Build history of the part. All positions in model axes, mm. A direction names the side the tool comes from. Round coordinates to 2 decimals unless told otherwise and drop trailing zeros. Write each loop counter-clockwise with the first axis right and the second up, starting at its lowest first coordinate (ties: lowest second). Pieces come first, ordered by that corner, then holes. Notation, with made-up numbers: (79.25, 43) - (137.25, 43) arc R29 cw to (137.25, 75) - close; hole circle Ø4 at (50.5, 83). An arc over 180 degrees is marked (long way). Answer as a JSON object with one key per item and string values. Group by question number.
Item 1: Slice it at C-C, the plane x = 49. List the corners of the cut face in (y, z).
Item 2: Slice it at B-B, the plane z = 36.22. List the corners of the cut face in (x, y).
Item 3: Slice it at A-A, the plane x = 10. List the corners of the cut face in (y, z).
Item 4: Slice it at D-D, the plane y = 21.75. List the corners of the cut face in (x, z), then the cut area to 4 significant figures.
Item 5: Probe line 1 (Z direction, x = 10, y = 10.75); line 2 (Z direction, x = 75.5, y = 4.75); line 3 (X direction, y = 27, z = -70). List the from-to ranges inside material, lowest first. Write a range as from..to.
Item 6: Which spindle directions (+Z, -Z, +X, -X, +Y, -Y) get a long thin tool onto all of the face, cutting with end or side? Do faces 4 (the flat face through (44, 15, 22)), 5 (the cylindrical face through (86.787, 3.252, -40.49)), 6 (the cylindrical face through (89.248, 15.21, -79.287)). Say none if no direction does.
Item 7: Flat gauge pins, fed straight in: pin 1 (7.5 mm diameter, centred on x = 36, y = 20, fed in from +Z); pin 2 (3 mm diameter, centred on x = 79, z = 14.5, fed in from +Y); pin 3 (5 mm diameter, centred on x = 56, z = -48.5, fed in from +Y). Where does each tip first touch, or does it go through?
Item 8: Two-plate mould, pull along Z, no slides. Class faces 1 (the flat face through (44, 16, -80)), 2 (the flat face through (0, 11, -32)), 3 (the cylindrical face through (45.56, 3.252, -76.787)): +Z half, -Z half, draft (parallel to the pull), parting line (faces both ways), or undercut.
from build123d import *

# Parameters (mm, degrees)
BOSS_EXTRUDE1_DEPTH    = 90
SHELL1_T               = -2.5
SKETCH2_W              = 90
SKETCH2_H              = 45
BOSS_EXTRUDE2_DEPTH    = 15
F_10_0MM_DOWEL_HOLE1_D = 10
FILLET1_R              = 2.5


with BuildPart() as part:
    # Sketch1 → Boss-Extrude1 (new body)
    with BuildSketch(Plane(origin=(0, 0, 0), x_dir=(0, 0, -1), z_dir=(1, 0, 0))):
        Polygon((0, 0), (80, 0), (80, 30), (0, 15), align=None)
    extrude(amount=BOSS_EXTRUDE1_DEPTH)

    # Shell1
    shell1_openings = [part.faces().sort_by_distance(p)[0] for p in [
        (45, 22.5, -40),
    ]]
    offset(amount=SHELL1_T, openings=shell1_openings, kind=Kind.INTERSECTION)

    # Sketch2 → Boss-Extrude2 (add)
    with BuildSketch(Plane.XZ):
        with Locations((45, 22.5)):
            Rectangle(SKETCH2_W, SKETCH2_H)
    extrude(amount=-BOSS_EXTRUDE2_DEPTH)

    # Ø10.0mm Dowel Hole1 (through all)
    with Locations(Plane.XZ):
        with Locations((10, 36.22)):
            Hole(F_10_0MM_DOWEL_HOLE1_D / 2)

    # Fillet1
    fillet1_edges = [part.edges().sort_by_distance(p)[0] for p in [
        (90, 15, -80),
        (2.5, 8.984375, -2.5),
        (2.5, 2.5, -40),
        (45, 2.5, -2.5),
        (2.5, 16.015625, -77.5),
        (45, 2.5, -77.5),
        (87.5, 8.984375, -2.5),
        (87.5, 2.5, -40),
        (87.5, 16.015625, -77.5),
        (45, 15, 45),
        (0, 7.5, 45),
        (90, 7.5, 45),
        (45, 0, 45),
        (0, 15, -80),
        (45, 0, -80),
    ]]
    fillet(fillet1_edges, radius=FILLET1_R)


solid = part.part
Geometry says:
{
 "1": {"outline": "(0, -77.5) arc R2.5 ccw to (2.5, -80) - (30, -80) - (29.53, -77.5) - (5, -77.5) arc R2.5 cw to (2.5, -75) - (2.5, -5) arc R2.5 cw to (5, -2.5) - (15.47, -2.5) - (15, 0) - (15, 42.5) arc R2.5 ccw to (12.5, 45) - (2.5, 45) arc R2.5 ccw to (0, 42.5) - close"},
 "2": {"outline": "(0, 0) - (5, 0) - (5, 15) - (0, 15) - close; (15, 0) - (90, 0) - (90, 15) - (15, 15) - close"},
 "3": {"outline": "(0, -77.5) arc R2.5 ccw to (2.5, -80) - (30, -80) - (29.53, -77.5) - (5, -77.5) arc R2.5 cw to (2.5, -75) - (2.5, -5) arc R2.5 cw to (5, -2.5) - (15.47, -2.5) - (15, 0) - (15, 31.22) - (0, 31.22) - close; (0, 41.22) - (15, 41.22) - (15, 42.5) arc R2.5 ccw to (12.5, 45) - (2.5, 45) arc R2.5 ccw to (0, 42.5) - close"},
 "4": {"outline": "(0, -77.5) arc R2.5 ccw to (2.5, -80) - (87.5, -80) arc R2.5 ccw to (90, -77.5) - (90, -36) - (87.5, -36) - (87.5, -75) arc R2.5 cw to (85, -77.5) - (5, -77.5) arc R2.5 cw to (2.5, -75) - (2.5, -36) - (0, -36) - close", "area": "432.5 mm^2"},
 "5": {"line 1": "z = -80..-77.5, -2.5..31.22, 41.22..45", "line 2": "z = -80..-77.49, -2.51..45", "line 3": "x = 0..2.5, 87.5..90"},
 "6": {"face 4": "+Z, +X, -X, +Y", "face 5": "+Y", "face 6": "-Z, +X, +Y, -Y"},
 "7": {"pin 1": "stops at z = -77.5", "pin 2": "stops at y = 15", "pin 3": "stops at y = 2.5"},
 "8": {"face 1": "-Z half", "face 2": "draft", "face 3": "undercut"}
}
